Autodesk Inventor part; units mm, degrees
ref_plane "YZ Plane" through (0, 0, 0) normal (1, 0, 0) x (0, 1, 0)
ref_plane "XZ Plane" through (0, 0, 0) normal (0, 1, 0) x (-1, 0, 0)
ref_plane "XY Plane" through (0, 0, 0) normal (0, 0, 1) x (1, 0, 0)
sketch "Esboço1" plane through (0, 0, 0) normal (0, 0, 1) x (1, 0, 0)
  line L0 (0, 8.6539) -> (150, 8.6539)
  line L1 (0, 8.6539) -> (0, 0.1539)
  line L2 (150, 8.6539) -> (150, 0.1539)
  line L3 (150, 0.1539) -> (150, 16.6456)
  line L4 (150, 8.6539) -> (270, 8.6539)
  line L5 (270, 8.6539) -> (285, 4.4039)
  line L6 (270, 0.1539) -> (285, 4.4039)
  line L7 (270, 0.1539) -> (0, 0.1539)
  line L8 (270, 8.6539) -> (270, 0.1539)
  dimension "d13" = 150
  dimension "d15" = 120
  dimension "d17" = 17
revolve "Revolução1" add sketch "Esboço1" angle 360 about axis through (270, 0.1539, 0) along (-1, 0, 0) contours L0 L2 L7 L1 | L4 L8 L7 L2
sketch "Esboço2" plane through (0, 0, 0) normal (0, 0, 1) x (1, 0, 0)
  line L0 (285, 0.1539) -> (315, 0.1539)
  line L1 (270, 8.6539) -> (270, -8.3461)
  line L2 (270, 0.1539) -> (285, 0.1539)
  line L3 (270, 8.6539) -> (270, 0.1539)
  line L4 (315, 0.1539) -> (270, 8.6539)
  point P0 (0, 0)
revolve "Revolução2" add sketch "Esboço2" angle 360 about axis through (285, 0.1539, 0) along (1, 0, 0)
sketch "Esboço3" plane through (0, 0, 0) normal (0, 1, 0) x (-1, 0, 0)
  line L0 (0, 0) -> (-25, 0)
  line L1 (0, -8.5) -> (0, 8.5)
  line L2 (0, 0) -> (-50, 0)
  line L3 (-50, 0) -> (-25, 0)
  line L4 (-50, 0) -> (-25, 0)
  line L5 (0, 0) -> (0, 21)
  line L6 (0, 21) -> (-14.7044, 0)
  line L7 (0, 21) -> (26.0415, 21) construction
  dimension "d54" = 21
  dimension "d57" = 125
sketch "Esboço4" plane through (0, 0, 0) normal (0, 1, 0) x (-1, 0, 0)
  line L0 (-270, -8.5) -> (-270, 8.5)
  line L1 (-134.6841, 0) -> (-134.6841, 21.5359)
  line L2 (-134.6841, 21.5359) -> (-147.3807, 0)
  line L3 (-134.6841, 0) -> (-147.3807, 0)
  point P0 (0, 0)
  dimension "d43" = 25
  dimension "d44" = 21.5359
extrude "Extrusão3" add sketch "Esboço4" along normal blind 3.5
pattern_circular "Padrão circular2" count 4 over 360 about axis through (135, 0.1539, 0) along (-1, 0, 0) of "Extrusão3"
sketch "Esboço5" plane through (0, 0.1539, 0) normal (-1, 0, 0) x (0, 0, 1)
  circle A0 centre (0, -0.1539) radius 5
  dimension "d50" = 10
extrude "Extrusão5" add sketch "Esboço3" along normal mid plane 3.5
pattern_circular "Padrão circular3" count 4 over 360 about axis through (135, 0.1539, 0) along (-1, 0, 0) of "Extrusão5"
extrude "Extrusão6" cut sketch "Esboço5" against normal blind 20
properties part number "120c"
Input: part model. Units: mm. Frame: model coordinates. A direction names the side the tool comes from. Coordinates: 2 decimals unless noted, no trailing zeros. Write each loop counter-clockwise with the first axis right and the second up, starting at its lowest first coordinate (ties: lowest second). Pieces come first, ordered by that corner, then holes.
1) Section C-C on x = 205. Output: boundary loops of the cut face in (y, z), and give its area (3 significant figures).
2) Pin query (flat end, axial travel): pin 1 Ø4.5 at (x, z) = (4.5, -13) entering from -Y; pin 2 Ø2.5 at (x, z) = (137.5, 14) entering from -Y; pin 3 Ø8.5 at (x, z) = (139, -17.5) entering from +Y. Return the tip coordinate at first contact, or that it passes through.
3) Section A-A on y = 15.5. Output: boundary loops of the cut face in (x, z), and give its area (3 significant figures).
4) Set-up query: faces 1 (the flat face through (3, 12, -1.596)), 2 (the flat face through (3, 12, 1.904)), 3 (the flat face through (137, 12, 0.154)), 4 (the flat face through (3, -1.442, -12)). Return all of +Z, -Z, +X, -X, +Y, -Y with unobstructed straight access to the full face (end or side cutting, diameter ignored); none if empty.
5) Material intervals for line 1 along Y through (x, z) = (12, 0); line 2 along Y through (x, z) = (7, 0); line 3 along Z through (x, y) = (104.5, 1.5), sorted ascending.
6) Mould query, pull axis X, two halves, no side actions, for faces 5 (the flat face through (4.39, -0.02, 14.73)), 6 (the flat face through (138.672, 14.925, -1.572)), 7 (the flat face through (137, 0, 12)). Classes: pulls with the +X half, pulls with the -X half, needs draft (parallel to the pull), parting line crosses it, or undercut.
7) Section B-B on z = 17. Output: boundary loops of the cut face in (x, y).
Check result:
1. outline: circle Ø17 at (0.15, 0)
1. area: 227 mm2
2. pin 1: stops at y = -1.44
2. pin 2: stops at y = 0
2. pin 3: stops at y = 0.31
3. outline: (0, -1.6) - (3.96, -1.6) - (3.96, 1.9) - (0, 1.9) - close; (134.68, -3.35) - (138.33, -3.35) - (138.33, 0.15) - (134.68, 0.15) - close
3. area: 26.6 mm2
4. face 1: -Z, -X, +Y
4. face 2: +Z, +X, -X, +Y
4. face 3: +Z, +X, +Y
4. face 4: -Z, -X, -Y
5. line 1: y = -8.35 to -5, 5 to 8.65
5. line 2: y = -10.85 to -5, 5 to 11.16
5. line 3: z = -8.39 to 8.39
6. face 5: undercut
6. face 6: pulls with the +X half
6. face 7: needs draft
7. outline: (0, -1.75) - (2.8, -1.75) - (2.8, 1.75) - (0, 1.75) - close; (134.68, 0) - (137.36, 0) - (137.36, 3.5) - (134.68, 3.5) - close
